from build123d import *

# Parameters (mm, degrees)
F0_W     = 304.8
F0_H     = 304.8
F1_DEPTH = 1.524
F2_W     = 72.39
F2_H     = 116.078
F3_DEPTH = 6.35
F4_R     = 44.45
F4_R_2   = 47.625
F5_DEPTH = 9.525


with BuildPart() as f1:
    # F0 (on Top) → F1 (new body)
    with BuildSketch(Plane.XY):
        Rectangle(F0_W, F0_H)
    extrude(amount=F1_DEPTH)

    # F2 (on face) → F3 (join)
    with BuildSketch(Plane.XY.offset(1.524)):
        with Locations((-55.245, 70.739)):
            Rectangle(F2_W, F2_H)
        with Locations((55.245, 70.739)):
            Rectangle(F2_W, F2_H)
        with Locations((-55.245, -70.739)):
            Rectangle(F2_W, F2_H)
        with Locations((55.245, -70.739)):
            Rectangle(F2_W, F2_H)
    extrude(amount=F3_DEPTH)

    # F4 (on face) → F5 (join)
    with BuildSketch(Plane.XY.offset(1.524)):
        with Locations((-55.245, 70.739)):
            Circle(F4_R)
        with Locations((55.245, 70.739)):
            Circle(F4_R)
        with Locations((-55.245, -70.739)):
            Circle(F4_R_2)
        with Locations((55.245, -70.739)):
            Circle(F4_R_2)
    extrude(amount=F5_DEPTH)


solid = f1.part
The listing builds one solid part. Answer for the finished solid, in the listing's coordinates (mm). A direction names the side the tool comes from. Coordinates: 2 decimals unless noted, no trailing zeros. Loops run counter-clockwise (first coordinate to the right, second up) from the corner with the lowest first, then second, coordinate; pieces in that order, holes last.
1) Find section A-A on z = 3.5. Give the number of separate pieces and of enclosed holes in the cut face, then the cut area to 3 significant figures.
2) A tool of negligible diameter and unlimited length cuts with its end or side. For faces 1 (the face through (55, -121, 7.874)), 2 (the face through (-14.184, 53.714, 7.278)), 3 (the face through (55, 71, 11.049)), 4 (the face through (55, 120, 7.874)), from which of +Z, -Z, +X, -X, +Y, -Y can it reach the whole face along a straight path? Write none if from no direction.
3) Find section C-C on y = 62. Write down the section's boundary in (x, z), then the cut area to 3 significant figures.
4) Find section D-D on x = -68. Write down the section's boundary in (y, z), then the cut area to 3 significant figures.
5) Flat-ended cylindrical pins translate along their axes: pin 1 Ø3 at (y, z) = (-25, 6.5) entering from +X; pin 2 Ø5 at (x, z) = (60, 5) entering from -Y; pin 3 Ø3 at (y, z) = (118.5, 4.5) entering from -X. Find the tip coordinate at first contact, or state that the pin passes through.
6) Find the intervals of material crossed by L1, parallel to X at y = 43, z = 4.75; L2, parallel to Y at x = -34, z = 3.75, in increasing order.
7) Find section B-B on x = 42.5. Write down the section's boundary in (y, z).
Values:
1. separate pieces: 4
1. enclosed holes: 0
1. area: 36,700 mm2
2. face 1: +Z, -Y
2. face 2: +Z
2. face 3: +Z, +X, -X, +Y, -Y
2. face 4: +Z, +Y
3. outline: (-152.4, 0) - (152.4, 0) - (152.4, 1.52) - (98.83, 1.52) - (98.83, 11.05) - (11.66, 11.05) - (11.66, 1.52) - (-11.66, 1.52) - (-11.66, 11.05) - (-98.83, 11.05) - (-98.83, 1.52) - (-152.4, 1.52) - close
3. area: 2,130 mm2
4. outline: (-152.4, 0) - (152.4, 0) - (152.4, 1.52) - (128.78, 1.52) - (128.78, 7.87) - (113.32, 7.87) - (113.32, 11.05) - (28.16, 11.05) - (28.16, 7.87) - (12.7, 7.87) - (12.7, 1.52) - (-12.7, 1.52) - (-12.7, 7.87) - (-24.85, 7.87) - (-24.85, 11.05) - (-116.62, 11.05) - (-116.62, 7.87) - (-128.78, 7.87) - (-128.78, 1.52) - (-152.4, 1.52) - close
4. area: 2,500 mm2
5. pin 1: stops at x = 91.44
5. pin 2: stops at y = -128.78
5. pin 3: stops at x = -91.44
6. L1: x = -91.44 to -19.05, 19.05 to 91.44
6. L2: y = -128.78 to -12.7, 12.7 to 128.78
7. outline: (-152.4, 0) - (152.4, 0) - (152.4, 1.52) - (128.78, 1.52) - (128.78, 7.87) - (113.32, 7.87) - (113.32, 11.05) - (28.16, 11.05) - (28.16, 7.87) - (12.7, 7.87) - (12.7, 1.52) - (-12.7, 1.52) - (-12.7, 7.87) - (-24.85, 7.87) - (-24.85, 11.05) - (-116.63, 11.05) - (-116.63, 7.87) - (-128.78, 7.87) - (-128.78, 1.52) - (-152.4, 1.52) - close
